Build history of the part. All positions in model axes, mm. A direction names the side the tool comes from. Give positions to 0.01 mm unless a question says otherwise; leave off trailing zeros. Loops run counter-clockwise (first coordinate to the right, second up) from the corner with the lowest first, then second, coordinate; pieces in that order, holes last.
1) Band-saw the part on A-A on x = 27.5. List the corners of the cut face in (y, z).
2) Band-saw the part on B-B on y = 42. List the corners of the cut face in (x, z).
3) Two-plate mould, pull along X, no slides. Class faces 4 (the flat face through (-103.754, 58.249, -5.07)), 5 (the flat face through (-29.824, 59, -5)), 6 (the flat face through (3, 57.235, -5)): +X half, -X half, draft (parallel to the pull), parting line (faces both ways), or undercut.
4) Band-saw the part on C-C on y = -43. List the corners of the cut face in (x, z).
5) Flat gauge pins, fed straight in: P1, Ø2, axis at y = -12, z = 1, coming from the +X side; P2, Ø4.5, axis at y = 60, z = -5, coming from the +X side; P3, Ø4.5, axis at y = 59.5, z = -6.5, coming from the -X side; P4, Ø0.5, axis at x = -13, z = 1, coming from the -Y side. Where does each tip first touch, or does it go through?
6) Band-saw the part on D-D on x = -88.5. List the corners of the cut face in (y, z), then the cut area to 3 significant figures.
7) 3-axis set-ups, long thin cutter, end or side, ignore diameter. For faces 1 (the cylindrical face through (-103.33, 60.67, -4.64)), 2 (the flat face through (-41.824, 59, -5)), 3 (the flat face through (-76, 57.235, -5)): which of +Z, -Z, +X, -X, +Y, -Y reach the whole face in a straight line?
8) Wall check: line 1 (Z direction, x = -16.5, y = 57); line 2 (Y direction, x = 14, z = -8.25); line 3 (X direction, y = -9, z = 1). Give the ranges that are in metal, low to high.
```python
from build123d import *

# Parameters (mm, degrees)
F1_DEPTH = 4
F2_W     = 67
F2_H     = 4
F3_DEPTH = 10
F4_R     = 3.3798989873
F5_R     = 2.1727922061
F6_SIZE  = 10
F7_R     = 2
F8_R     = 2


with BuildPart() as f1:
    # F0 (on Top) → F1 (new body)
    with BuildSketch(Plane.XY):
        Polygon((37.1763631701, 61.2354552448), (-108.8236368299, 61.2354552448), (-108.8236368299, 36.2354552448), (-108.8236368299, -55.7645447552), (-82.8236368299, -55.7645447552), (-82.8236368299, 36.2354552448), (37.1763631701, 36.2354552448), align=None)
    extrude(amount=F1_DEPTH)

    # F2 (on face) → F3 (join)
    with BuildSketch(Plane(origin=(0, 0, 0), x_dir=(1, 0, 0), z_dir=(0, 0, -1))):
        with Locations((3.6763631701, -59.2354552448)):
            Rectangle(F2_W, F2_H)
        with Locations((-75.3236368299, -59.2354552448)):
            Rectangle(F2_W, F2_H)
    extrude(amount=F3_DEPTH)

    # F4
    f4_edges = [f1.edges().sort_by_distance(p)[0] for p in [
        (-82.823637, 36.235455, 2),
    ]]
    fillet(f4_edges, radius=F4_R)

    # F5
    f5_edges = [f1.edges().sort_by_distance(p)[0] for p in [
        (-82.823637, -11.454494, 4),
        (-21.133687, 36.235455, 4),
    ]]
    fillet(f5_edges, radius=F5_R)

    # F6
    f6_edges = [f1.edges().sort_by_distance(p)[0] for p in [
        (-108.823637, 59.235455, -10),
    ]]
    chamfer(f6_edges, length=F6_SIZE)

    # F7
    f7_edges = [f1.edges().sort_by_distance(p)[0] for p in [
        (-103.823637, 61.235455, -5),
        (-35.823637, 61.235455, 4),
        (-108.823637, 2.735455, 4),
        (-108.823637, 61.235455, 2),
        (37.176363, 61.235455, -3),
        (3.676363, 61.235455, -10),
        (-70.323637, 61.235455, -10),
        (37.176363, 49.821851, 4),
    ]]
    fillet(f7_edges, radius=F7_R)

    # F8
    f8_edges = [f1.edges().sort_by_distance(p)[0] for p in [
        (-95.910033, -55.764545, 4),
    ]]
    fillet(f8_edges, radius=F8_R)


solid = f1.part
```
Findings below:
1. outline: (36.24, 0) - (57.24, 0) - (57.24, -10) - (59.24, -10) arc R2 ccw to (61.24, -8) - (61.24, 2) arc R2 ccw to (59.24, 4) - (38.41, 4) arc R2.17 ccw to (36.24, 1.83) - close
2. outline: (-108.82, 0) - (37.18, 0) - (37.18, 2) arc R2 ccw to (35.18, 4) - (-106.82, 4) arc R2 ccw to (-108.82, 2) - close
3. face 4: -X half
3. face 5: undercut
3. face 6: draft
4. outline: (-108.82, 0) - (-82.82, 0) - (-82.82, 1.83) arc R2.17 ccw to (-85, 4) - (-106.82, 4) arc R2 ccw to (-108.82, 2) - close
5. P1: stops at x = -82.82
5. P2: stops at x = 37.18
5. P3: stops at x = -104.56
5. P4: stops at y = 36.24
6. outline: (-55.76, 0) - (57.24, 0) - (57.24, -10) - (59.24, -10) arc R2 ccw to (61.24, -8) - (61.24, 2) arc R2 ccw to (59.24, 4) - (-53.76, 4) arc R2 ccw to (-55.76, 2) - close
6. area: 505 mm2
7. face 1: -Z, -X, +Y
7. face 2: -Z, +Y, -Y
7. face 3: -Z, +X, -X, -Y
8. line 1: z = 0 to 4
8. line 2: y = 57.24 to 61.22
8. line 3: x = -108.82 to -82.82
